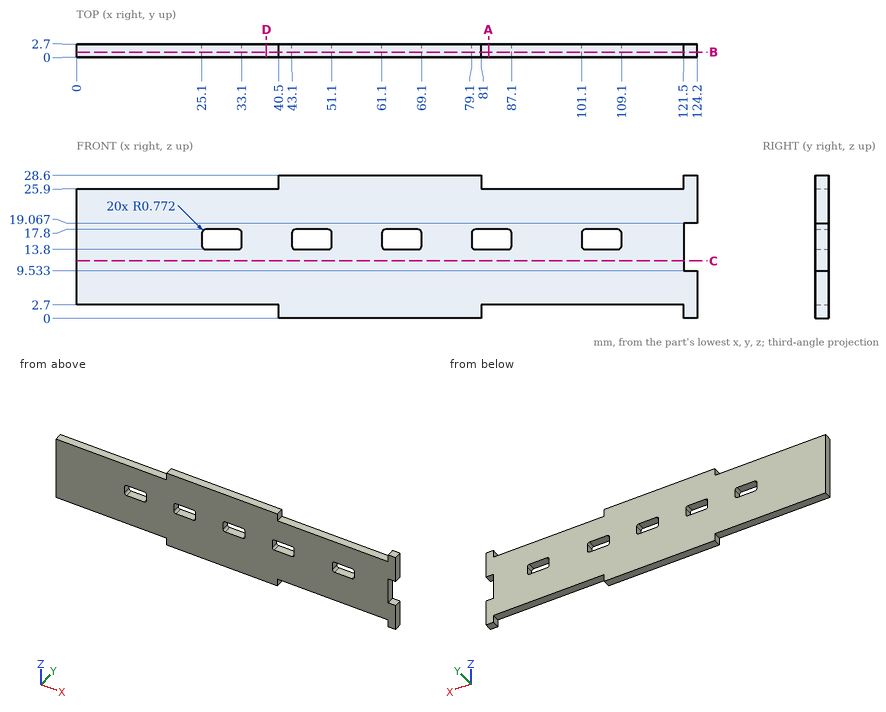
Print and shaded views of the part. All mm, measured from the part's lowest x, y and z. Round coordinates to 2 decimals unless told otherwise and drop trailing zeros. Order: outer loops, then holes, each group sorted by start corner. A loop starts at its lowest first (then second) coordinate and runs counter-clockwise, first axis right, second up.
Q1. Wall check: L1, parallel to X at y = 1.5, z = 17; L2, parallel to X at y = 1.6, z = 14 (1 decimal); L3, parallel to X at y = 1.3, z = 27.5. Give the ranges that are in metal, low to high.
Q2. Drop flat-ended pins along their axis: pin 1 (1.4 mm diameter, centred on y = 1.5, z = 16.5, fed in from +X); pin 2 (1.3 mm diameter, centred on y = 2, z = 27.5, fed in from -X); pin 3 (0.7 mm diameter, centred on y = 1, z = 16, fed in from -X); pin 4 (1.4 mm diameter, centred on x = 106, y = 2, fed in from -Z). Give the stop position or say it passes through.
Q3. Slice it at D-D (x = 38). Write the cut outline in (y, z).
Q4. Slice it at A-A (x = 82.5). Write the cut outline in (y, z).
Q5. Slice it at C-C (z = 11.5). Write the cut outline in (x, y), and give its area (3 significant figures).
Q6. Slice it at B-B (y = 1.05). State how many separate pieces and enclosed holes the cut face has, and give its area (3 significant figures).
Results below:
1. L1: x = 0 to 25.1, 33.1 to 43.1, 51.1 to 61.1, 69.1 to 79.1, 87.1 to 101.1, 109.1 to 121.5
1. L2: x = 0 to 25.4, 32.8 to 43.4, 50.8 to 61.4, 68.8 to 79.4, 86.8 to 101.4, 108.8 to 121.5
1. L3: x = 40.5 to 81, 121.5 to 124.2
2. pin 1: stops at x = 121.5
2. pin 2: stops at x = 40.5
2. pin 3: stops at x = 0
2. pin 4: stops at z = 2.7
3. outline: (0, 2.7) - (2.7, 2.7) - (2.7, 25.9) - (0, 25.9) - close
4. outline: (0, 2.7) - (2.7, 2.7) - (2.7, 13.8) - (0, 13.8) - close; (0, 17.8) - (2.7, 17.8) - (2.7, 25.9) - (0, 25.9) - close
5. outline: (0, 0) - (121.5, 0) - (121.5, 2.7) - (0, 2.7) - close
5. area: 328 mm2
6. separate pieces: 1
6. enclosed holes: 5
6. area: 2,930 mm2
